```python
from build123d import *

# Parameters (mm, degrees)
F0_R     = 23.5061904225
F1_DEPTH = 6.35
F2_R     = 21.5857863289
F2_R_2   = 19.0486454652
F3_DEPTH = 15.24
F4_R     = 5.08


# Not quite as in the source:
# - a fillet or chamfer that OpenCascade refuses, or shapes differently, is made with other operations: its cross-section is extruded or revolved along the edge and cut away or added


with BuildPart() as f1:
    # F0 (on Top) → F1 (new body)
    with BuildSketch(Plane.XY):
        Circle(F0_R)
    extrude(amount=F1_DEPTH)

    # F2 (on Top) → F3 (join)
    with BuildSketch(Plane.XY):
        Circle(F2_R)
        Circle(F2_R_2, mode=Mode.SUBTRACT)
    extrude(amount=F3_DEPTH)

    # F4
    f4_edges = [f1.edges().sort_by_distance(p)[0] for p in [
        (-23.50619, 0, 0),
    ]]
    fillet(f4_edges, radius=F4_R)

    # F5: chamfer of 2.54 on 1 edges, made by hand

    # F5_s1 → F5_t2 (revolve, cut)
    with BuildSketch(Plane.XZ):
        Polygon((21.5857863289, 12.7), (19.0457863289, 15.24), (21.5857863289, 15.24), align=None)
    revolve(axis=Axis((0, 0, 15.24), (0, 0, 1)), mode=Mode.SUBTRACT)


solid = f1.part
```
Design review of the part built by this model. Coordinates are the model's own, in mm. A direction names the side the tool comes from. Give positions to 0.01 mm unless a question says otherwise; leave off trailing zeros. Write each loop counter-clockwise with the first axis right and the second up, starting at its lowest first coordinate (ties: lowest second). Pieces come first, ordered by that corner, then holes. Notation, with made-up numbers: (14.5, -15.75) - (45.5, -15.75) arc R23 cw to (45.5, 6.25) - close; hole circle Ø3 at (-39.75, -32.5). An arc over 180 degrees is marked (long way). Return JSON: item names as keys, results as strings. Group by question number.
(1) To check wall thickness, follow probe 1 along Y at (x, z) = (0, 10); probe 2 along Z at (x, y) = (-9.5, -7). State the ranges of each line that lie inside material, in increasing order.
(2) We need section A-A, the plane y = 0. Give the boundary of the cut face in (x, z), then the cut area to 3 significant figures.
(3) Mouldability with a two-part tool opening along Y and no side actions: class faces 1 (the cylindrical face through (-2.48, 18.887, 10.731)), 2 (the cylindrical face through (-5, -21, 9)), 3 (the flat face through (0, 0, 0)) as +Y half, -Y half, draft (parallel to the pull), parting line (faces both ways), or undercut.
(4) Insertion check: pin 1 (4 mm diameter, centred on x = 7, z = 3, fed in from -Y); pin 2 (2 mm diameter, centred on x = -18, z = 7, fed in from -Y); pin 3 (8 mm diameter, centred on x = -3, y = 7, fed in from +Z). Each pin has a flat end and moves straight along its axis. Give the tip position at first contact, or say it passes through.
(5) Machinability: for faces 4 (the cylindrical face through (-5.096, -22.947, 5.706)), 5 (the flat face through (7, -21, 6.35)), which of the approach directions +Z, -Z, +X, -X, +Y, -Y give a long, thin tool a straight path to every point of the face, cutting with its end or side? Answer none if there is none.
(6) We need section D-D, the plane z = 3.5. Give the boundary of the cut face in (x, y), then the cut area to 3 significant figures.
(7) We need section C-C, the plane z = 9.75. Give the boundary of the cut face in (x, y).
Reported:
{
 "1": {"probe 1": "y = -21.59 to -19.05, 19.05 to 21.59", "probe 2": "z = 0 to 6.35"},
 "2": {"outline": "(-23.51, 5.08) arc R5.08 ccw to (-18.43, 0) - (18.43, 0) arc R5.08 ccw to (23.51, 5.08) - (23.51, 6.35) - (21.59, 6.35) - (21.59, 12.7) - (19.05, 15.24) - (19.05, 6.35) - (-19.05, 6.35) - (-19.05, 15.24) - (-21.59, 12.7) - (-21.59, 6.35) - (-23.51, 6.35) - close", "area": "326 mm2"},
 "3": {"face 1": "undercut", "face 2": "parting line", "face 3": "draft"},
 "4": {"pin 1": "stops at y = -22.8", "pin 2": "stops at y = -15.98", "pin 3": "stops at z = 6.35"},
 "5": {"face 4": "+Z, -Z", "face 5": "+Z"},
 "6": {"outline": "circle Ø46.51 at (0, 0)", "area": "1,700 mm2"},
 "7": {"outline": "circle Ø43.17 at (0, 0); hole circle Ø38.1 at (0, 0)"}
}
